Input: part model. Units: mm. Frame: model coordinates. A direction names the side the tool comes from. Coordinates: 2 decimals unless noted, no trailing zeros. Order: outer loops, then holes, each group sorted by start corner. A loop starts at its lowest first (then second) coordinate and runs counter-clockwise, first axis right, second up. Notation, with made-up numbers: (61.25, -15.75) -> (83.25, -15.75) arc R32 cw to (83.25, 15.25) -> close; hole circle Ø7 at (88, 88). An arc over 180 degrees is marked (long way). Use CSV: the item, a comma, the result in double quotes. Start each with the question number.
```python
from build123d import *

# Parameters (mm, degrees)
SKETCH_1_R          = 8.75
SKETCH_1_R_2        = 8.25
EXTRUDE_2_DEPTH     = 10
SKETCH_2_R          = 8.25
SKETCH_2_R_2        = 2
EXTRUDE_3_DEPTH     = 4
EXTRUDE_4_DEPTH     = 8
SKETCH_5_W          = 3
SKETCH_5_H          = 8
EXTRUDE_5_DEPTH     = 3
SKETCH_6_W          = 3
SKETCH_6_H          = 8
EXTRUDE_6_DEPTH     = 3
SKETCH_7_R          = 1.5
CUT_EXTRUDE_1_DEPTH = 3
FILLET_1_R          = 5
FILLET_3_R          = 2
SKETCH_8_R          = 8.75
SKETCH_8_R_2        = 8.25
EXTRUDE_7_DEPTH     = 8
SKETCH_9_R          = 8.25
SKETCH_9_R_2        = 6
EXTRUDE_8_DEPTH     = 2
EXTRUDE_9_DEPTH     = 8
SKETCH_11_R         = 1.5
CUT_EXTRUDE_2_DEPTH = 8
CUT_EXTRUDE_3_DEPTH = 8
CUT_EXTRUDE_4_DEPTH = 8
SKETCH_14_R         = 8.75
SKETCH_14_R_2       = 8.25
EXTRUDE_10_DEPTH    = 8
EXTRUDE_11_DEPTH    = 8
SKETCH_16_R         = 1.5
CUT_EXTRUDE_5_DEPTH = 8
CUT_EXTRUDE_6_DEPTH = 10
CUT_EXTRUDE_7_DEPTH = 10


with BuildPart() as part:
    # 草图1 → 凸台-拉伸2 (new body)
    with BuildSketch(Plane(origin=(0, 0, 0), x_dir=(1, 0, 0), z_dir=(0, 1, 0))):
        Circle(SKETCH_1_R)
        Circle(SKETCH_1_R_2, mode=Mode.SUBTRACT)
    extrude(amount=EXTRUDE_2_DEPTH)

    # 草图2 → 凸台-拉伸3 (add)
    with BuildSketch(Plane(origin=(0, 0, 0), x_dir=(1, 0, 0), z_dir=(0, 1, 0))):
        Circle(SKETCH_2_R)
        Circle(SKETCH_2_R_2, mode=Mode.SUBTRACT)
    extrude(amount=EXTRUDE_3_DEPTH)

    # 草图3 → 凸台-拉伸4 (add)
    with BuildSketch(Plane(origin=(0, 0, 0), x_dir=(1, 0, 0), z_dir=(0, 1, 0))):
        Polygon((-2, 8.518362519), (2, 8.518362519), (2, 15), (15, 15), (15, 18), (2, 18), (-2, 18), (-15, 18), (-15, 15), (-2, 15), align=None)
    extrude(amount=EXTRUDE_4_DEPTH)

    # 草图5 → 凸台-拉伸5 (add)
    with BuildSketch(Plane(origin=(15, 0, 0), x_dir=(0, 0, -1), z_dir=(1, 0, 0))):
        with Locations((16.5, 4)):
            Rectangle(SKETCH_5_W, SKETCH_5_H)
    extrude(amount=EXTRUDE_5_DEPTH)

    # 草图6 → 凸台-拉伸6 (add)
    with BuildSketch(Plane.ZY.offset(15)):
        with Locations((-16.5, 4)):
            Rectangle(SKETCH_6_W, SKETCH_6_H)
    extrude(amount=EXTRUDE_6_DEPTH)

    # 草图7 → 切除-拉伸1 (cut)
    with BuildSketch(Plane(origin=(0, 0, -18), x_dir=(-1, 0, 0), z_dir=(0, 0, -1))):
        with Locations((-15, 3.754021035)):
            Circle(SKETCH_7_R)
    cut_extrude_1 = extrude(amount=-CUT_EXTRUDE_1_DEPTH, mode=Mode.SUBTRACT)

    # 镜向1: 切除-拉伸1 across plane
    add(cut_extrude_1.mirror(Plane(origin=(0, 0, 0), x_dir=(0, 0, 1), z_dir=(1, 0, 0))), mode=Mode.SUBTRACT)

    # 圆角1
    fillet_1_edges = [part.edges().sort_by_distance(p)[0] for p in [
        (-2, 4, -8.518362519),
        (2, 4, -8.518362519),
    ]]
    fillet(fillet_1_edges, radius=FILLET_1_R)

    # 圆角3
    fillet_3_edges = [part.edges().sort_by_distance(p)[0] for p in [
        (-2, 4, -15),
        (2, 4, -15),
    ]]
    fillet(fillet_3_edges, radius=FILLET_3_R)

    # 草图17 → 切除-拉伸6 (cut)
    with BuildSketch(Plane(origin=(0, 0, 0), x_dir=(1, 0, 0), z_dir=(0, 1, 0))):
        Polygon((-27.724622817, 21.69601187), (-7.349237756, -14.338233932), (7.177657148, -11.696980313), (13.592130223, 5.659829184), (24.157144699, 16.036182687), (2.467165325, 27.553795746), (0, 27.553795746), align=None)
    extrude(amount=CUT_EXTRUDE_6_DEPTH, mode=Mode.SUBTRACT)


with BuildPart() as body_2:
    # 草图8 → 凸台-拉伸7 (new body)
    with BuildSketch(Plane(origin=(0, 0, 0), x_dir=(1, 0, 0), z_dir=(0, 1, 0))):
        with Locations((27.184954533, 0)):
            Circle(SKETCH_8_R)
        with Locations((27.184954533, 0)):
            Circle(SKETCH_8_R_2, mode=Mode.SUBTRACT)
    extrude(amount=EXTRUDE_7_DEPTH)

    # 草图9 → 凸台-拉伸8 (add)
    with BuildSketch(Plane.XZ):
        with Locations((27.184954533, 0)):
            Circle(SKETCH_9_R)
        with Locations((27.184954533, 0)):
            Circle(SKETCH_9_R_2, mode=Mode.SUBTRACT)
    extrude(amount=-EXTRUDE_8_DEPTH)

    # 草图10 → 凸台-拉伸9 (add)
    with BuildSketch(Plane(origin=(0, 0, 0), x_dir=(1, 0, 0), z_dir=(0, 1, 0))):
        Polygon((27.184954533, -18), (45.184954533, -18), (45.184954533, -14.663867829), (29.184954533, -14.663867829), (29.184954533, -8.518362519), (25.184954533, -8.518362519), (25.184954533, -14.663867829), (9.184954533, -14.663867829), (9.184954533, -18), align=None)
    extrude(amount=EXTRUDE_9_DEPTH)

    # 草图11 → 切除-拉伸2 (cut)
    with BuildSketch(Plane.XY.offset(18)):
        with Locations((12.184954533, 4)):
            Circle(SKETCH_11_R)
        with Locations((42.184954533, 4)):
            Circle(SKETCH_11_R)
    extrude(amount=-CUT_EXTRUDE_2_DEPTH, mode=Mode.SUBTRACT)

    # 草图12 → 切除-拉伸3 (cut)
    with BuildSketch(Plane.XY.offset(18)):
        with BuildLine():
            Line((10.684954533, 4), (10.684954533, 5))
            ThreePointArc((10.684954533, 5), (12.184954533, 6.5), (13.684954533, 5))
            Line((13.684954533, 5), (13.684954533, 4))
            Line((13.684954533, 4), (13.684954533, 3))
            ThreePointArc((13.684954533, 3), (12.184954533, 1.5), (10.684954533, 3))
            Line((10.684954533, 3), (10.684954533, 4))
        make_face()
    extrude(amount=-CUT_EXTRUDE_3_DEPTH, mode=Mode.SUBTRACT)

    # 草图13 → 切除-拉伸4 (cut)
    with BuildSketch(Plane.XY.offset(18)):
        with BuildLine():
            Line((40.684954533, 4), (40.684954533, 5))
            ThreePointArc((40.684954533, 5), (42.184954533, 6.5), (43.684954533, 5))
            Line((43.684954533, 5), (43.684954533, 4))
            Line((43.684954533, 4), (43.684954533, 3))
            ThreePointArc((43.684954533, 3), (42.184954533, 1.5), (40.684954533, 3))
            Line((40.684954533, 3), (40.684954533, 4))
        make_face()
    extrude(amount=-CUT_EXTRUDE_4_DEPTH, mode=Mode.SUBTRACT)


with BuildPart() as body_3:
    # 草图14 → 凸台-拉伸10 (new body)
    with BuildSketch(Plane(origin=(0, 0, 0), x_dir=(1, 0, 0), z_dir=(0, 1, 0))):
        with Locations((-35.091635024, 0)):
            Circle(SKETCH_14_R)
        with Locations((-35.091635024, 0)):
            Circle(SKETCH_14_R_2, mode=Mode.SUBTRACT)
    extrude(amount=EXTRUDE_10_DEPTH)

    # 草图15 → 凸台-拉伸11 (add)
    with BuildSketch(Plane(origin=(0, 0, 0), x_dir=(1, 0, 0), z_dir=(0, 1, 0))):
        Polygon((-37.091635024, -15), (-37.091635024, -8.518362519), (-33.091635024, -8.518362519), (-33.091635024, -15), (-17.091635024, -15), (-17.091635024, -18), (-53.091635024, -18), (-53.091635024, -15), align=None)
    extrude(amount=EXTRUDE_11_DEPTH)

    # 草图16 → 切除-拉伸5 (cut)
    with BuildSketch(Plane.XY.offset(18)):
        with Locations((-50.091635024, 4)):
            Circle(SKETCH_16_R)
        with Locations((-20.091635024, 4)):
            Circle(SKETCH_16_R)
    extrude(amount=-CUT_EXTRUDE_5_DEPTH, mode=Mode.SUBTRACT)

    # 草图18 → 切除-拉伸7 (cut)
    with BuildSketch(Plane(origin=(0, 0, 0), x_dir=(1, 0, 0), z_dir=(0, 1, 0))):
        Polygon((-5.334341173, 26.542566247), (-7.107938045, -29.653340051), (-79.00930818, -22.653952159), (-79.00930818, -19.085416228), (-48.199741002, 26.542566247), align=None)
    extrude(amount=CUT_EXTRUDE_7_DEPTH, mode=Mode.SUBTRACT)


solid = body_2.part
```
1. Access query for faces 4 (the face through (29.185, 4, 12)), 5 (the face through (12.2, 1.5, 16.4)), 6 (the face through (35.054, 4.958, -2.478)). Directions: +Z, -Z, +X, -X, +Y, -Y. A direction counts if a zero-diameter tool reaches every point of the face in a straight line with its end or side. Return the directions, or none.
2. Material intervals for line 1 along Z through (x, y) = (33.5, 2.75); line 2 along Z through (x, y) = (32.5, 7.75); line 3 along X through (y, z) = (5.75, 16.25), sorted ascending.
3. Pull-direction query (X, two-part tool) for faces 1 (the face through (27, 4, 18)), 2 (the face through (25.185, 4, 12)), 3 (the face through (31, 2, -5)); classes: released by +X, released by -X, zero draft, split by the parting line, or undercut.
4. Section C-C on y = 7. Return loops of the section in (x, z).
5. Contact query for flat-ended pins moving along their axis: P1, Ø3, axis at x = 40.5, y = 6.5, coming from the -Z side; P2, Ø1, axis at y = 4, z = 12, coming from the -X side; P3, Ø2, axis at x = 18.5, y = 2.5, coming from the -Z side. Output: stop coordinate, or through.
6. Section D-D on z = -7. Return loops of the section in (x, y).
7. Section A-A on y = 4. Return loops of the section in (x, z), then the cut area to 3 significant figures.
8. Section B-B on z = 0. Return loops of the section in (x, y), then the cut area to 3 significant figures.
Values follow:
1,face 4,"+X, +Y, -Y"
1,face 5,"+Z, -Z"
1,face 6,"+Y"
2,line 1,"z = -6.06 to -5.31, 5.31 to 6.06, 14.66 to 18"
2,line 2,"z = -6.95 to -6.31, 6.31 to 6.95, 14.66 to 18"
2,line 3,"x = 9.18 to 10.89, 13.48 to 40.89, 43.48 to 45.18"
3,face 1,"zero draft"
3,face 2,"released by -X"
3,face 3,"undercut"
4,outline,"(9.18, 14.66) -> (25.18, 14.66) -> (25.18, 8.52) arc R8.75 ccw (long way) to (29.18, 8.52) -> (29.18, 14.66) -> (45.18, 14.66) -> (45.18, 18) -> (9.18, 18) -> close; hole circle Ø16.5 at (27.18, 0)"
5,P1,"stops at z = 14.66"
5,P2,"stops at x = 25.18"
5,P3,"stops at z = -4.18"
6,outline,"(21.93, 0) -> (32.43, 0) -> (32.43, 8) -> (31.55, 8) -> (31.55, 2) -> (22.82, 2) -> (22.82, 8) -> (21.93, 8) -> close"
7,outline,"(9.18, 14.66) -> (10.68, 14.66) -> (10.68, 18) -> (9.18, 18) -> close; (13.68, 14.66) -> (25.18, 14.66) -> (25.18, 8.52) arc R8.75 ccw (long way) to (29.18, 8.52) -> (29.18, 14.66) -> (40.68, 14.66) -> (40.68, 18) -> (13.68, 18) -> close; (43.68, 14.66) -> (45.18, 14.66) -> (45.18, 18) -> (43.68, 18) -> close; hole circle Ø16.5 at (27.18, 0)"
7,area,"151 mm2"
8,outline,"(18.43, 0) -> (21.18, 0) -> (21.18, 2) -> (18.93, 2) -> (18.93, 8) -> (18.43, 8) -> close; (33.18, 0) -> (35.93, 0) -> (35.93, 8) -> (35.43, 8) -> (35.43, 2) -> (33.18, 2) -> close"
8,area,"17.0 mm2"
